```python
from build123d import *

# Parameters (mm, degrees)
F0_W        = 56
F0_H        = 76
F1_DEPTH    = 10
F2_D        = 9.525
F3_T1_DEPTH = 150.1699053678
F4_R        = 5
F5_D        = 8


# Not quite as in the source:
# - a fillet or chamfer that OpenCascade refuses, or shapes differently, is made with other operations: its cross-section is extruded or revolved along the edge and cut away or added
# - a length typed as a fraction of an inch, garbled in the dataset ("3 / 203.2 mm" for 3/8 in), is restored


with BuildPart() as f1:
    # F0 (on Top) → F1 (new body)
    with BuildSketch(Plane.XY):
        Rectangle(F0_W, F0_H)
        Polygon((-31, 18), (-28, -38), (-28, 38), (-31, 38), align=None)
        Polygon((28, 38), (28, -38), (31, 18), (31, 38), align=None)
    extrude(amount=-F1_DEPTH)

    # F2 (through all)
    with Locations(Plane.XY):
        with Locations((0, -22)):
            Hole(F2_D / 2)

    # F3: fillet of radius 29.576 on 2 edges, made by hand

    # F3_s2 → F3_t1 (cut)
    with BuildSketch(Plane.XY.offset(-80.0849526839)):
        with BuildLine():
            ThreePointArc((-0.0339810736, -38), (20.3123431081, -29.889480854), (29.4996700065, -10.0061598793))
            Line((29.4996700065, -10.0061598793), (28, -38))
            Line((28, -38), (-0.0339810736, -38))
        make_face()
        with BuildLine():
            ThreePointArc((0.0339810736, -38), (-20.3123431081, -29.889480854), (-29.4996700065, -10.0061598793))
            Line((-29.4996700065, -10.0061598793), (-28, -38))
            Line((-28, -38), (0.0339810736, -38))
        make_face()
    extrude(amount=F3_T1_DEPTH, mode=Mode.SUBTRACT)

    # F4
    f4_edges = [f1.edges().sort_by_distance(p)[0] for p in [
        (-31, 38, -5),
        (31, 38, -5),
    ]]
    fillet(f4_edges, radius=F4_R)

    # F5 (through all)
    with Locations(Plane.XY):
        with Locations((-19, 28), (19, 28)):
            Hole(F5_D / 2)


solid = f1.part
```
The listing builds one solid part. Answer for the finished solid, in the listing's coordinates (mm). Give positions to 0.01 mm unless a question says otherwise; leave off trailing zeros. Loops run counter-clockwise (first coordinate to the right, second up) from the corner with the lowest first, then second, coordinate; pieces in that order, holes last. Notation, with made-up numbers: (-13, -19) - (-4, -19) arc R26 ccw to (-4, 15) - close; hole circle Ø1 at (30.5, 10). An arc over 180 degrees is marked (long way). Return JSON: item names as keys, results as strings. Group by question number.
1. Find section B-B (z = -8.25). Write down the section's boundary in (x, y) (1 decimal), then the cut area to 3 significant figures.
2. Find section C-C (x = 19). Write down the section's boundary in (y, z).
3. Straight lines are drawn through the part: line 1 (X direction, y = 27.5, z = -7.25); line 2 (Y direction, x = 0, z = -6.5); line 3 (Y direction, x = -19, z = -3). For each, find the intervals that lie inside material, in ascending order. Write a range as [from, to].
4. Find section D-D (y = -20). Write down the section's boundary in (x, z).
5. Given pin 1 Ø6 at (y, z) = (0, -5.5) entering from +X; pin 2 Ø4 at (x, z) = (-21.5, -6.5) entering from -Y; pin 3 Ø1.5 at (x, y) = (22, -13.5) entering from +Z; pin 4 Ø5 at (x, y) = (19, 28) entering from +Z, each flat-ended and moving along its own axis, determine where each tip first touches the part or whether it passes through.
6. Determine the mould class of faces 1 (the cylindrical face through (1.03, -26.65, -5.07)), 2 (the flat face through (30.24, 3.8, -4.93)), 3 (the flat face through (31, 25, -5)) for opening direction Y: pulls with the +Y half, pulls with the -Y half, needs draft (parallel to the pull), parting line crosses it, or undercut.
7. Find section A-A (y = 28). Write down the section's boundary in (x, z).
Verdict:
{
 "1": {"outline": "(-31, 18) - (-29.5, -10) arc R29.6 ccw to (0, -38) arc R29.6 ccw to (29.5, -10) - (31, 18) - (31, 33) arc R5 ccw to (26, 38) - (-26, 38) arc R5 ccw to (-31, 33) - close; hole circle Ø8 at (-19, 28); hole circle Ø9.5 at (0, -22); hole circle Ø8 at (19, 28)", "area": "4,030 mm^2"},
 "2": {"outline": "(-31.06, -10) - (24, -10) - (24, 0) - (-31.06, 0) - close; (32, -10) - (38, -10) - (38, 0) - (32, 0) - close"},
 "3": {"line 1": "x = [-31, -22.97], [-15.03, 15.03], [22.97, 31]", "line 2": "y = [-38, -26.76], [-17.24, 38]", "line 3": "y = [-31.06, 24], [32, 38]"},
 "4": {"outline": "(-27.18, -10) - (-4.32, -10) - (-4.32, 0) - (-27.18, 0) - close; (4.32, -10) - (27.18, -10) - (27.18, 0) - (4.32, 0) - close"},
 "5": {"pin 1": "stops at x = 30.2", "pin 2": "stops at y = -30.63", "pin 3": "stops at z = 0", "pin 4": "passes through"},
 "6": {"face 1": "undercut", "face 2": "pulls with the -Y half", "face 3": "needs draft"},
 "7": {"outline": "(-31, -10) - (-23, -10) - (-23, 0) - (-31, 0) - close; (-15, -10) - (15, -10) - (15, 0) - (-15, 0) - close; (23, -10) - (31, -10) - (31, 0) - (23, 0) - close"}
}
